CAD build for the part. Positions are in the model's coordinates, mm. A direction names the side the tool comes from. Round coordinates to 2 decimals unless told otherwise and drop trailing zeros. Order: outer loops, then holes, each group sorted by start corner. A loop starts at its lowest first (then second) coordinate and runs counter-clockwise, first axis right, second up. Notation, with made-up numbers: M -26,85.5 L -4,85.5 A18 ccw -4,101.5 Z; hole C -24,-7 d2. An arc over 180 degrees is marked long. Put each result on its own line as item: value.
```python
from build123d import *

# Parameters (mm, degrees)
EXTRUDE_1_DEPTH     = 4
SKETCH_2_R          = 11.5
EXTRUDE_2_DEPTH     = 9
SKETCH_3_W          = 8.5
SKETCH_3_H          = 8.5
CUT_EXTRUDE_1_DEPTH = 10


with BuildPart() as part:
    # Эскиз1 → Бобышка-Вытянуть1 (new body)
    with BuildSketch(Plane.XY):
        with BuildLine():
            Line((-44.5, 8), (44.5, 8))
            ThreePointArc((44.5, 8), (52.5, 0), (44.5, -8))
            Line((44.5, -8), (-44.5, -8))
            ThreePointArc((-44.5, -8), (-52.5, 0), (-44.5, 8))
        make_face()
    extrude(amount=EXTRUDE_1_DEPTH)

    # Эскиз2 → Бобышка-Вытянуть2 (add)
    with BuildSketch(Plane(origin=(0, 0, 0), x_dir=(-1, 0, 0), z_dir=(0, 0, -1))):
        Circle(SKETCH_2_R)
    extrude(amount=-EXTRUDE_2_DEPTH)

    # Эскиз3 → Вырез-Вытянуть1 (cut, through all)
    with BuildSketch(Plane(origin=(0, 0, 0), x_dir=(-1, 0, 0), z_dir=(0, 0, -1))):
        Rectangle(SKETCH_3_W, SKETCH_3_H)
    extrude(amount=-CUT_EXTRUDE_1_DEPTH, mode=Mode.SUBTRACT)


solid = part.part
```
Item 1: Probe line 1 along Z through (x, y) = (29, 6); line 2 along X through (y, z) = (-3.25, 8.25); line 3 along Y through (x, z) = (-41.5, 1). List the from-to ranges inside material, lowest first. Write a range as [from, to].
Answers below:
line 1: [0, 4]
line 2: [-11.03, -4.25], [4.25, 11.03]
line 3: [-8, 8]
Item 2: Band-saw the part on A-A on x = 0. Give the cut face in (y, z), and give its area (4 significant figures).
Answers below:
outline: M -11.5,0 L -4.25,0 L -4.25,9 L -11.5,9 Z; M 4.25,0 L 11.5,0 L 11.5,9 L 4.25,9 Z
area: 130.5 mm²
Item 3: Band-saw the part on B-B on y = 0. Give the cut face in (x, z), and give its area (4 significant figures).
Answers below:
outline: M -52.5,0 L -4.25,0 L -4.25,9 L -11.5,9 L -11.5,4 L -52.5,4 Z; M 4.25,0 L 52.5,0 L 52.5,4 L 11.5,4 L 11.5,9 L 4.25,9 Z
area: 458.5 mm²
Item 4: Mould opens along Y. For faces 4 (the flat face through (1, 5, 0)), 5 (the flat face through (-27, 8, 2)), 6 (the flat face through (4.25, 0, 4)) say: pulls with the +Y half, pulls with the -Y half, needs draft (parallel to the pull), parting line crosses it, or undercut.
Answers below:
face 4: needs draft
face 5: pulls with the +Y half
face 6: undercut
Item 5: Band-saw the part on C-C on z = 1. Give the cut face in (x, y), and give its area (3 significant figures).
Answers below:
outline: M -44.5,-8 L -8.26,-8 A11.5 ccw 8.26,-8 L 44.5,-8 A8 ccw 44.5,8 L 8.26,8 A11.5 ccw -8.26,8 L -44.5,8 A8 ccw Z; hole M -4.25,-4.25 L 4.25,-4.25 L 4.25,4.25 L -4.25,4.25 Z
area: 1,630 mm²
Item 6: Tool access for faces 1 (the flat face through (27, -8, 2)), 2 (the flat face through (26, 8, 2)), 3 (the cylindrical face through (-10.97, 3.45, 5.44)): list every direction of +Z, -Z, +X, -X, +Y, -Y with a clear straight run to the whole face (end or side of a thin tool).
Answers below:
face 1: +Z, -Z, +X, -Y
face 2: +Z, -Z, +X, +Y
face 3: +Z
Item 7: Band-saw the part on D-D on y = 7. Give the cut face in (x, z), and give its area (3 significant figures).
Answers below:
outline: M -48.37,0 L 48.37,0 L 48.37,4 L 9.12,4 L 9.12,9 L -9.12,9 L -9.12,4 L -48.37,4 Z
area: 478 mm²
Item 8: Pin check, flat tips, straight feed: P1, Ø4.5, axis at x = -30.5, z = 2.5, coming from the +Y side; P2, Ø4, axis at x = -41.5, y = -5.5, coming from the +Z side; P3, Ø10, axis at x = -14, y = 6.5, coming from the +Z side; P4, Ø4.5, axis at x = 25, z = 2, coming from the -Y side. Stop position of each tip, or through.
Answers below:
P1: y = 8
P2: z = 4
P3: z = 9
P4: y = -8
